Work out the finished part from the listing and answer in its coordinate system (mm). A direction names the side the tool comes from. Give positions to 0.01 mm unless a question says otherwise; leave off trailing zeros. Write each loop counter-clockwise with the first axis right and the second up, starting at its lowest first coordinate (ties: lowest second). Pieces come first, ordered by that corner, then holes.
1) Given pin 1 Ø1.5 at (x, z) = (-16.5, -3) entering from -Y, flat-ended and moving along its own axis, determine where the tip first touches the part or whether it passes through.
2) A tool of negligible diameter and unlimited length cuts with its end or side. For faces 1 (the face through (0, 3.302, 0)), 2 (the face through (-7.008, -0.313, 0.353)), from which of +Z, -Z, +X, -X, +Y, -Y can it reach the whole face along a straight path? Write none if from no direction.
3) Find section B-B (x = -13). Determine the outline of the cut face in (y, z) (3 decimals).
4) Find section A-A (z = 0). Determine the outline of the cut face in (x, y) (3 decimals).
5) Find section D-D (x = 15). Determine the outline of the cut face in (y, z).
6) A straight line is drawn through the part: probe 1 along Y at (x, z) = (-19, 3). Find the intervals that lie inside material, in ascending order.
7) Find section C-C (z = 1.75). Determine the outline of the cut face in (x, y) (3 decimals).
8) Determine the mould class of faces 3 (the face through (0, 2, 5.08)), 4 (the face through (-20.955, 2, 0)), 5 (the face through (9.213, -0.313, -0.45)) for opening direction X: pulls with the +X half, pulls with the -X half, needs draft (parallel to the pull), parting line crosses it, or undercut.
```python
from build123d import *

# Parameters (mm, degrees)
SKETCH1_W           = 41.91
SKETCH1_H           = 10.16
BOSS_EXTRUDE1_DEPTH = 3.302
SKETCH2_R           = 1.174037675
BOSS_EXTRUDE2_DEPTH = 0.635


with BuildPart() as part:
    # Sketch1 → Boss-Extrude1 (new body)
    with BuildSketch(Plane(origin=(0, 0, 0), x_dir=(1, 0, 0), z_dir=(0, 1, 0))):
        Rectangle(SKETCH1_W, SKETCH1_H)
    extrude(amount=BOSS_EXTRUDE1_DEPTH)

    # Sketch2 → Boss-Extrude2 (add)
    with BuildSketch(Plane.XZ):
        with Locations((-13.462, 0)):
            Circle(SKETCH2_R)
        with Locations((-8.128, 0)):
            Circle(SKETCH2_R)
        with Locations((8.128, 0)):
            Circle(SKETCH2_R)
        with Locations((13.462, 0)):
            Circle(SKETCH2_R)
    extrude(amount=BOSS_EXTRUDE2_DEPTH)


solid = part.part
```
Results:
1. pin 1: stops at y = 0
2. face 1: +Z, -Z, +X, -X, +Y
2. face 2: -Y
3. outline: (-0.635, -1.079) - (0, -1.079) - (0, -5.08) - (3.302, -5.08) - (3.302, 5.08) - (0, 5.08) - (0, 1.079) - (-0.635, 1.079) - close
4. outline: (-20.955, 0) - (-14.636, 0) - (-14.636, -0.635) - (-12.288, -0.635) - (-12.288, 0) - (-9.302, 0) - (-9.302, -0.635) - (-6.954, -0.635) - (-6.954, 0) - (6.954, 0) - (6.954, -0.635) - (9.302, -0.635) - (9.302, 0) - (12.288, 0) - (12.288, -0.635) - (14.636, -0.635) - (14.636, 0) - (20.955, 0) - (20.955, 3.302) - (-20.955, 3.302) - close
5. outline: (0, -5.08) - (3.3, -5.08) - (3.3, 5.08) - (0, 5.08) - close
6. probe 1: y = 0 to 3.3
7. outline: (-20.955, 0) - (20.955, 0) - (20.955, 3.302) - (-20.955, 3.302) - close
8. face 3: needs draft
8. face 4: pulls with the -X half
8. face 5: undercut
